CAD build for the part. Positions are in the model's coordinates, mm. A direction names the side the tool comes from. Round coordinates to 2 decimals unless told otherwise and drop trailing zeros. Order: outer loops, then holes, each group sorted by start corner. A loop starts at its lowest first (then second) coordinate and runs counter-clockwise, first axis right, second up.
```python
from build123d import *

# Parameters (mm, degrees)
F0_W     = 53.975
F0_H     = 31.115
F1_DEPTH = 3.175
F2_R     = 3.17499
F3_W     = 50.165
F3_H     = 27.305
F3_W_2   = 47.625
F3_H_2   = 24.765
F4_DEPTH = 3.175
F6_D     = 5.08


# Not quite as in the source:
# - a fillet or chamfer is up to 0.001 mm smaller than in the source, because OpenCascade refuses the exact size


with BuildPart() as f1:
    # F0 (on Top) → F1 (new body)
    with BuildSketch(Plane.XY):
        Rectangle(F0_W, F0_H)
    extrude(amount=F1_DEPTH)

    # F2 (radius 3.175 in the source; OpenCascade refuses exactly that, so slightly less here)
    f2_edges = [f1.edges().sort_by_distance(p)[0] for p in [
        (0, -15.5575, 3.175),
        (-26.9875, 0, 3.175),
        (0, 15.5575, 3.175),
        (26.9875, 0, 3.175),
        (26.9875, -15.5575, 1.5875),
        (26.9875, 15.5575, 1.5875),
        (-26.9875, 15.5575, 1.5875),
        (-26.9875, -15.5575, 1.5875),
    ]]
    fillet(f2_edges, radius=F2_R)

    # F3 (on face) → F4 (join)
    with BuildSketch(Plane(origin=(0, 0, 0), x_dir=(1, 0, 0), z_dir=(0, 0, -1))):
        Rectangle(F3_W, F3_H)
        Rectangle(F3_W_2, F3_H_2, mode=Mode.SUBTRACT)
    extrude(amount=F4_DEPTH)

    # F6 (through all)
    with Locations(Plane.XY.offset(3.175)):
        with Locations((-7.9375, 0), (2.2225, 0), (12.3825, 0)):
            Hole(F6_D / 2)


solid = f1.part
```
1. Tool access for faces 1 (the face through (23.812, 0, -2)), 2 (the face through (25.082, 0, -2)), 3 (the face through (0, 13.652, -2)), 4 (the face through (0, -13.652, -2)), 5 (the face through (-25.082, 0, -2)): list every direction of +Z, -Z, +X, -X, +Y, -Y with a clear straight run to the whole face (end or side of a thin tool).
2. Cut at C-C, the plane z = -2. Write the cut outline in (x, y), and give its area (3 significant figures).
3. Drill centre lines: line 1 (X direction, y = 8.5, z = -0.5); line 2 (Y direction, x = 16, z = -1); line 3 (Z direction, x = 1.5, y = 3.5) (3 decimals). Where is each one in solid material? Low to high.
4. Mould opens along Y. For faces 6 (the face through (-10.36, 0.76, 1.57)), 7 (the face through (26.1, 0.2, 2.2)), 8 (the face through (0.33, 14.65, 2.22)), 9 (the face through (4.09, 1.72, 1.57)) say: released by +Y, released by -Y, zero draft, split by the parting line, or undercut.
5. Pin check, flat tips, straight feed: P1, Ø3, axis at x = -7.94, y = 0, coming from the -Z side; P2, Ø2, axis at x = -1, y = 0, coming from the -Z side; P3, Ø1.6, axis at y = -2, z = -2, coming from the +X side; P4, Ø1.6, axis at y = -6, z = -1.5, coming from the -X side. Stop position of each tip, or through.
6. Cut at D-D, the plane z = 1. Write the cut outline in (x, y), and give its area (3 significant figures).
7. Cut at A-A, the plane y = 0. Give the number of separate pieces and of enclosed holes in the cut face, and give its area (3 significant figures).
Outcome:
1. face 1: -Z
1. face 2: -Z, +X, +Y, -Y
1. face 3: -Z, +X, -X, +Y
1. face 4: -Z, +X, -X, -Y
1. face 5: -Z, -X, +Y, -Y
2. outline: (-25.08, -13.65) - (25.08, -13.65) - (25.08, 13.65) - (-25.08, 13.65) - close; hole (-23.81, -12.38) - (23.81, -12.38) - (23.81, 12.38) - (-23.81, 12.38) - close
2. area: 190 mm2
3. line 1: x = -25.08 to -23.81, 23.81 to 25.08
3. line 2: y = -13.65 to -12.38, 12.38 to 13.65
3. line 3: z = 0 to 3.175
4. face 6: undercut
4. face 7: zero draft
4. face 8: released by +Y
4. face 9: undercut
5. P1: passes through
5. P2: stops at z = 0
5. P3: stops at x = 25.08
5. P4: stops at x = -25.08
6. outline: (-26.83, -12.38) arc R3.01 ccw to (-23.81, -15.4) - (23.81, -15.4) arc R3.01 ccw to (26.83, -12.38) - (26.83, 12.38) arc R3.01 ccw to (23.81, 15.4) - (-23.81, 15.4) arc R3.01 ccw to (-26.83, 12.38) - close; hole circle Ø5.08 at (-7.94, 0); hole circle Ø5.08 at (2.22, 0); hole circle Ø5.08 at (12.38, 0)
6. area: 1,580 mm2
7. separate pieces: 4
7. enclosed holes: 0
7. area: 127 mm2
